Source: three-view drawing plus pictorial views. Frame: mm from the lowest corner of the part. A direction names the side the tool comes from. Give positions to 0.01 mm unless a question says otherwise; leave off trailing zeros. Order: outer loops, then holes, each group sorted by start corner. A loop starts at its lowest first (then second) coordinate and runs counter-clockwise, first axis right, second up. Notation, with made-up numbers: (-32, 4) - (-19, 4) arc R21 cw to (-19, 40) - close; hole circle Ø5 at (-11.5, 3.5). An arc over 180 degrees is marked (long way). Answer in a Markdown table with one row per item. Add a question column.
1. Section query C-C on x = 30.5. Return loops of the section in (y, z).
2. Section query D-D on y = 17. Return loops of the section in (x, z) (3 decimals), and give its area (3 significant figures).
3. Access query for the marked faces 4, 5 and 6. Directions: +Z, -Z, +X, -X, +Y, -Y. A direction counts if a zero-diameter tool reaches every point of the face in a straight line with its end or side. Return the directions, or none.
4. Contact query for flat-ended pins moving along their axis: pin 1 (1 mm diameter, centred on x = 18.5, y = 17.5, fed in from +Z); pin 2 (1 mm diameter, centred on y = 16.5, z = 1, fed in from -X); pin 3 (1.5 mm diameter, centred on x = 6, z = 6, fed in from -Y) (3 decimals); pin 4 (2.5 mm diameter, centred on x = 6, z = 5, fed in from +Y) (3 decimals). Output: stop coordinate, or through.
5. Section query B-B on y = 7.75. Return loops of the section in (x, z) (3 decimals).
6. Ray query, line 1 (Y direction, x = 29.5, z = 4.25); line 2 (X direction, y = 22, z = 11.75); line 3 (X direction, y = 7.75, z = 11.25). Return the intervals inside material, ascending. Write a range as [from, to].
7. Mould query, pull axis X, two halves, no side actions, for the marked faces 1, 2 and 3. Classes: released by +X, released by -X, zero draft, split by the parting line, or undercut.
8. Section query A-A on z = 11. Return loops of the section in (x, y) (3 decimals).
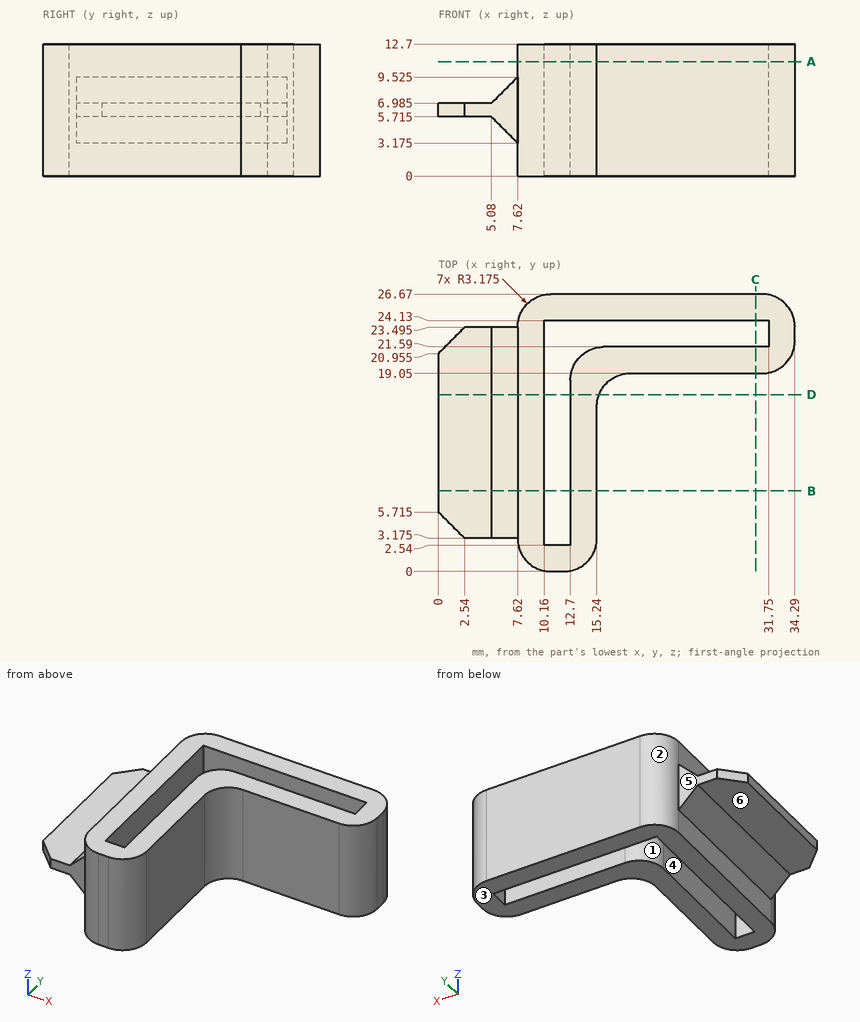
Answer:
| question | item | result |
|---|---|---|
| 1 | outline | (19.05, 0) - (21.59, 0) - (21.59, 12.7) - (19.05, 12.7) - close; (24.13, 0) - (26.67, 0) - (26.67, 12.7) - (24.13, 12.7) - close |
| 2 | outline | (0, 5.715) - (5.08, 5.715) - (7.62, 3.175) - (7.62, 0) - (10.16, 0) - (10.16, 12.7) - (7.62, 12.7) - (7.62, 9.525) - (5.08, 6.985) - (0, 6.985) - close; (12.7, 0) - (15.446, 0) - (15.446, 12.7) - (12.7, 12.7) - close |
| 2 | area | 83.3 mm² |
| 3 | face 4 | +Z, -Z |
| 3 | face 5 | +Z, -Z, -X, +Y |
| 3 | face 6 | -Z, -X, +Y, -Y |
| 4 | pin 1 | passes through |
| 4 | pin 2 | stops at x = 7.62 |
| 4 | pin 3 | stops at y = 3.175 |
| 4 | pin 4 | stops at y = 23.495 |
| 5 | outline | (0, 5.715) - (5.08, 5.715) - (7.62, 3.175) - (7.62, 0) - (10.16, 0) - (10.16, 12.7) - (7.62, 12.7) - (7.62, 9.525) - (5.08, 6.985) - (0, 6.985) - close; (12.7, 0) - (15.24, 0) - (15.24, 12.7) - (12.7, 12.7) - close |
| 6 | line 1 | y = [19.05, 21.59], [24.13, 26.67] |
| 6 | line 2 | x = [7.62, 10.16], [31.75, 34.28] |
| 6 | line 3 | x = [7.62, 10.16], [12.7, 15.24] |
| 7 | face 1 | undercut |
| 7 | face 2 | released by -X |
| 7 | face 3 | zero draft |
| 8 | outline | (7.62, 3.175) arc R3.175 ccw to (10.795, 0) - (12.065, 0) arc R3.175 ccw to (15.24, 3.175) - (15.24, 15.875) arc R3.175 cw to (18.415, 19.05) - (31.115, 19.05) arc R3.175 ccw to (34.29, 22.225) - (34.29, 23.495) arc R3.175 ccw to (31.115, 26.67) - (10.795, 26.67) arc R3.175 ccw to (7.62, 23.495) - close; hole (10.16, 2.54) - (12.7, 2.54) - (12.7, 18.415) arc R3.175 cw to (15.875, 21.59) - (31.75, 21.59) - (31.75, 24.13) - (10.16, 24.13) - close |
